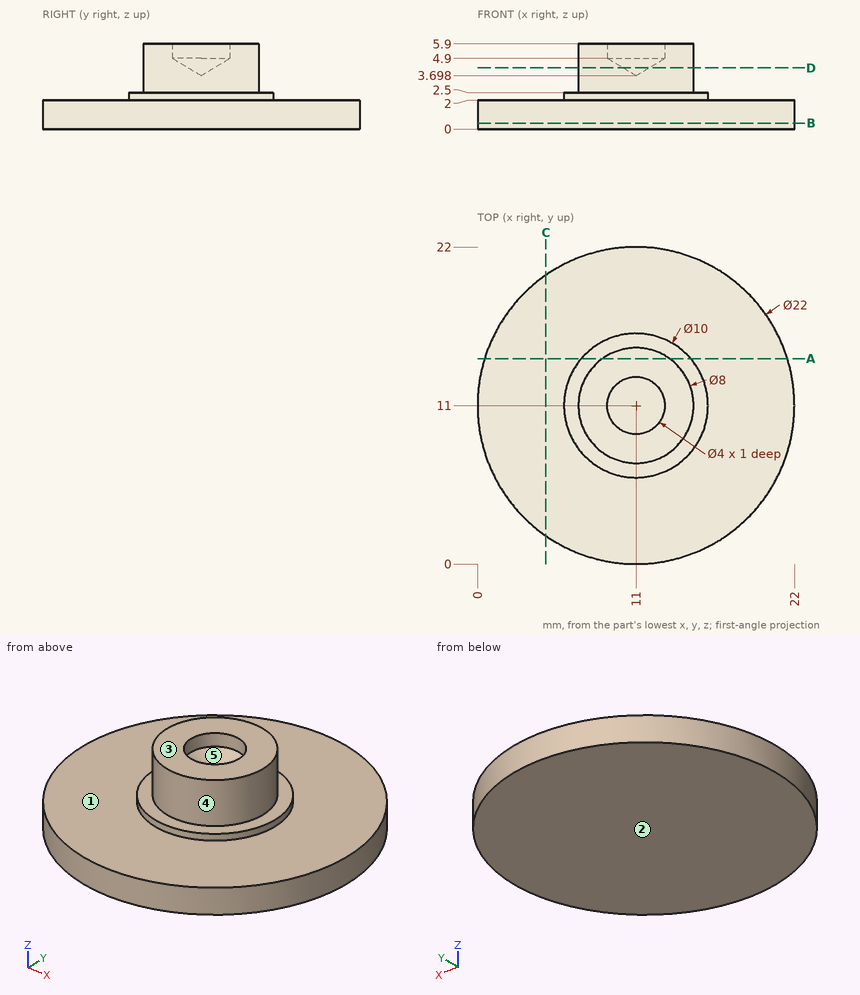
Verification items for this drawing (mm, ordinates from the low corner). A direction names the side the tool comes from. Give positions to 0.01 mm unless a question says otherwise; leave off trailing zeros. Loops run counter-clockwise (first coordinate to the right, second up) from the corner with the lowest first, then second, coordinate; pieces in that order, holes last. Notation, with made-up numbers: M 77,40 L 103,40 A13 ccw 103,46 Z; hole C -29.75,61.5 d6. An arc over 180 degrees is marked long. Return JSON: item names as keys, results as strings. Group by question number.
1. Mould release check, pull along X, two halves, no side actions. Record for the marked faces 3, 4 and 5: released by +X, released by -X, zero draft, split by the parting line, or undercut.
2. Cross-section at D-D on z = 4.25. Record the boundary of the cut face in (x, y), plus the area to 3 significant figures.
3. Cross-section at C-C on x = 4.75. Record the boundary of the cut face in (y, z), plus the area to 3 significant figures.
4. Go/stop test with flat-tipped pins: pin 1 (1.5 mm diameter, centred on x = 6.5, z = 0.5, fed in from +Y); pin 2 (5 mm diameter, centred on x = 12, y = 19, fed in from +Z). Record where each tip stops, or that it passes through.
5. Cross-section at B-B on z = 0.4. Record the boundary of the cut face in (x, y), plus the area to 3 significant figures.
6. Cross-section at A-A on y = 14.25. Record the boundary of the cut face in (x, z).
7. Tool access check on the marked faces 1 and 2. Record the directions out of +Z, -Z, +X, -X, +Y, -Y that give a thin tool (end or side, any length) a straight path to the whole face; none if there is none.
8. Thickness scan on L1, parallel to Y at x = 11, z = 5.4; L2, parallel to Z at x = 3, y = 15.25; L3, parallel to X at y = 7.75, z = 0.5. Record the ranges inside material, lowest first.
Return value:
{
 "1": {"face 3": "zero draft", "face 4": "split by the parting line", "face 5": "undercut"},
 "2": {"outline": "C 11,11 d8; hole C 11,11 d1.84", "area": "47.6 mm^2"},
 "3": {"outline": "M 1.95,0 L 20.05,0 L 20.05,2 L 1.95,2 Z", "area": "36.2 mm^2"},
 "4": {"pin 1": "y = 21.34", "pin 2": "z = 2"},
 "5": {"outline": "C 11,11 d22", "area": "380 mm^2"},
 "6": {"outline": "M 0.49,0 L 21.51,0 L 21.51,2 L 14.8,2 L 14.8,2.5 L 13.33,2.5 L 13.33,5.9 L 8.67,5.9 L 8.67,2.5 L 7.2,2.5 L 7.2,2 L 0.49,2 Z"},
 "7": {"face 1": "+Z", "face 2": "-Z, +X, -X, +Y, -Y"},
 "8": {"L1": "7 to 9, 13 to 15", "L2": "0 to 2", "L3": "0.49 to 21.51"}
}
